Model file for the job. Use its own axes, mm. A direction names the side the tool comes from. Round coordinates to 2 decimals unless told otherwise and drop trailing zeros. Loops run counter-clockwise (first coordinate to the right, second up) from the corner with the lowest first, then second, coordinate; pieces in that order, holes last. Notation, with made-up numbers: M -25,30.25 L -10,30.25 A11 ccw -10,40.25 Z; hole C 22,33 d11. An arc over 180 degrees is marked long. Use a Markdown table: item, result. Add a question column.
Q1. Cut at D-D (x = -249.5). Give the cut face in (y, z), plus the area to 3 significant figures.
Q2. Mould opens along Z. For faces 1 (the face through (320.06, 51.24, 19.23)), 2 (the face through (29, 38, 0)), 3 (the face through (337.055, 50.384, 19.269)), 4 (the face through (29, 38, 39)) say: +Z half, -Z half, draft (parallel to the pull), parting line (faces both ways), or undercut.
Q3. Cut at B-B (x = 25). Give the cut face in (y, z).
Q4. Pin check, flat tips, straight feed: pin 1 (19.5 mm diameter, centred on x = -142.5, z = 24, fed in from +Y); pin 2 (1.5 mm diameter, centred on y = 63.5, z = 24, fed in from -X); pin 3 (1.5 mm diameter, centred on y = 27.5, z = 10, fed in from +X); pin 4 (3 mm diameter, centred on x = 10, y = 72, fed in from +Z). Stop position of each tip, or through.
Q5. Cut at A-A (z = 11). Give the cut face in (x, y), plus the area to 3 significant figures.
Q6. Tool access for faces 5 (the face through (-55, 37, 19)), 6 (the face through (323.06, 51.31, 19.27)), 7 (the face through (157, 62, 19)): list every direction of +Z, -Z, +X, -X, +Y, -Y with a clear straight run to the whole face (end or side of a thin tool).
Q7. Probe line 1 (Y direction, x = 10, z = 2.15); line 2 (Y direction, x = -337, z = 19); line 3 (Z direction, x = -387, y = 33.5). List the from-to ranges inside material, lowest first. Write a range as from..to.
Q8. Cut at C-C (y = 51). Give the cut face in (x, z).
from build123d import *

# Parameters (mm, degrees)
BOSS_EXTRUDE1_DEPTH = 39
SHELL1_T            = -3
SKETCH2_W           = 33
SKETCH2_H           = 14
CUT_EXTRUDE1_DEPTH  = 455.896372
SKETCH3_R           = 2.5
CUT_EXTRUDE2_DEPTH  = 456.047881521


with BuildPart() as part:
    # Sketch1 → Boss-Extrude1 (new body)
    with BuildSketch(Plane.XY):
        with BuildLine():
            Line((309.062127233, 40), (-425.902299809, 40))
            Line((-425.902299809, 40), (-445.896371903, 26))
            Line((-445.896371903, 26), (-445.896371903, 20))
            Line((-445.896371903, 20), (309.062127233, 20))
            ThreePointArc((309.062127233, 20), (340.062127233, 51), (309.062127233, 82))
            Line((309.062127233, 82), (10, 82))
            ThreePointArc((10, 82), (0, 72), (10, 62))
            Line((10, 62), (309.062127233, 62))
            ThreePointArc((309.062127233, 62), (320.062127233, 51), (309.062127233, 40))
        make_face()
    extrude(amount=BOSS_EXTRUDE1_DEPTH)

    # Shell1
    shell1_openings = [part.faces().sort_by_distance(p)[0] for p in [
        (-435.899335856, 33, 19.5),
    ]]
    offset(amount=SHELL1_T, openings=shell1_openings, kind=Kind.INTERSECTION)

    # Sketch2 → Cut-Extrude1 (cut)
    with BuildSketch(Plane.ZY.offset(445.896371903)):
        with Locations((19.5, 72)):
            Rectangle(SKETCH2_W, SKETCH2_H)
        with Locations((19.5, 30)):
            Rectangle(SKETCH2_W, SKETCH2_H)
    extrude(amount=-CUT_EXTRUDE1_DEPTH, mode=Mode.SUBTRACT)

    # Sketch3 → Cut-Extrude2 (cut, through all)
    with BuildSketch(Plane.XY.offset(39)):
        with Locations((10, 72)):
            Circle(SKETCH3_R)
    extrude(amount=-CUT_EXTRUDE2_DEPTH, mode=Mode.SUBTRACT)


solid = part.part
Checked values:
| question | item | result |
|---|---|---|
| 1 | outline | M 20,0 L 40,0 L 40,39 L 20,39 Z; hole M 23,3 L 37,3 L 37,36 L 23,36 Z |
| 1 | area | 318 mm^2 |
| 2 | face 1 | draft |
| 2 | face 2 | -Z half |
| 2 | face 3 | undercut |
| 2 | face 4 | +Z half |
| 3 | outline | M 20,0 L 40,0 L 40,39 L 20,39 Z; M 62,0 L 82,0 L 82,39 L 62,39 Z; hole M 23,3 L 37,3 L 37,36 L 23,36 Z; hole M 65,3 L 79,3 L 79,36 L 65,36 Z |
| 4 | pin 1 | stops at y = 40 |
| 4 | pin 2 | stops at x = 3.68 |
| 4 | pin 3 | stops at x = 330.12 |
| 4 | pin 4 | passes through |
| 5 | outline | M -445.9,20 L 309.06,20 A31 ccw 309.06,82 L 10,82 A10 ccw 2.86,79 L 309.06,79 A28 cw 309.06,23 L -445.9,23 Z; M -430.19,37 L 309.06,37 A14 ccw 309.06,65 L 2.86,65 A10 ccw 10,62 L 309.06,62 A11 cw 309.06,40 L -425.9,40 Z |
| 5 | area | 6,700 mm^2 |
| 6 | face 5 | -X |
| 6 | face 6 | none |
| 6 | face 7 | +Z, -Z, -X |
| 7 | line 1 | y = 20..40, 62..69.5, 74.5..82 |
| 7 | line 2 | y = 20..23, 37..40 |
| 7 | line 3 | z = 0..3, 36..39 |
| 8 | outline | M 320.06,0 L 340.06,0 L 340.06,39 L 320.06,39 Z; hole M 323.06,3 L 337.06,3 L 337.06,36 L 323.06,36 Z |
